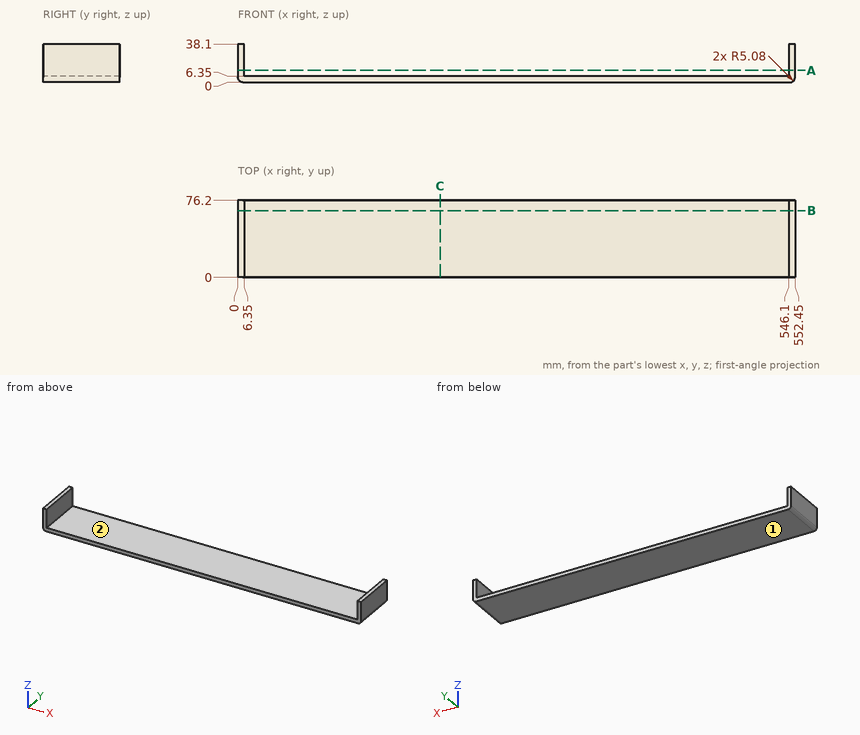
Drawing for the job (mm, zero at the part's lowest x, y, z). Round coordinates to 2 decimals unless told otherwise and drop trailing zeros. Loops run counter-clockwise (first coordinate to the right, second up) from the corner with the lowest first, then second, coordinate; pieces in that order, holes last. Notation, with made-up numbers: (55, -14) -> (72, -14) arc R27 cw to (72, 2) -> close; hole circle Ø6 at (-2, 15). An arc over 180 degrees is marked (long way). Answer as CSV lines item,"result". Start each with the question number.
1) Mould opens along X. For the marked faces 1 and 2 say: +X half, -X half, draft (parallel to the pull), parting line (faces both ways), or undercut.
2) Slice it at A-A (z = 12). List the corners of the cut face in (x, y).
3) Slice it at C-C (x = 200.5). List the corners of the cut face in (y, z).
4) Probe line 1 along X through (y, z) = (39, 12.5); line 2 along Z through (x, y) = (206.5, 19); line 3 along X through (y, z) = (50, 5). List the from-to ranges inside material, lowest first.
5) Pin check, flat tips, straight feed: P1, Ø12, axis at x = 179, z = 15, coming from the +Y side; P2, Ø16, axis at y = 44, z = 20, coming from the -X side. Stop position of each tip, or through.
6) Slice it at B-B (y = 66). List the corners of the cut face in (x, z).
Filled in:
1,face 1,"draft"
1,face 2,"undercut"
2,outline,"(0, 0) -> (6.35, 0) -> (6.35, 76.2) -> (0, 76.2) -> close; (546.1, 0) -> (552.45, 0) -> (552.45, 76.2) -> (546.1, 76.2) -> close"
3,outline,"(0, 0) -> (76.2, 0) -> (76.2, 6.35) -> (0, 6.35) -> close"
4,line 1,"x = 0 to 6.35, 546.1 to 552.45"
4,line 2,"z = 0 to 6.35"
4,line 3,"x = 0 to 552.45"
5,P1,"passes through"
5,P2,"stops at x = 0"
6,outline,"(0, 5.08) arc R5.08 ccw to (5.08, 0) -> (547.37, 0) arc R5.08 ccw to (552.45, 5.08) -> (552.45, 38.1) -> (546.1, 38.1) -> (546.1, 6.35) -> (6.35, 6.35) -> (6.35, 38.1) -> (0, 38.1) -> close"
